Design review of the part built by this model. Coordinates are the model's own, in mm. Face numbers are marked on the shaded views. A direction names the side the tool comes from. Coordinates: 2 decimals unless noted, no trailing zeros. Order: outer loops, then holes, each group sorted by start corner. A loop starts at its lowest first (then second) coordinate and runs counter-clockwise, first axis right, second up. Notation, with made-up numbers: M -7,-19.5 L 9,-19.5 A22 ccw 9,-12.5 Z; hole C 48,-19 d7. An arc over 180 degrees is marked long. Answer as a JSON object with one key per item and string values.
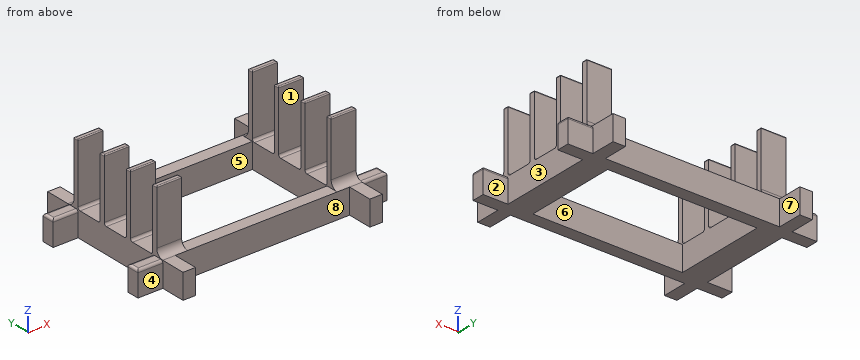
from build123d import *

# Parameters (mm, degrees)
SKETCH2_W           = 37
SKETCH2_H           = 60
BOSS_EXTRUDE1_DEPTH = 10
SKETCH3_W           = 10
SKETCH3_H           = 2
BOSS_EXTRUDE2_DEPTH = 25
FILLET1_R           = 3
FILLET2_R           = 3
FILLET3_R           = 1
FILLET6_START       = -11
FILLET6_DEPTH       = 11
FILLET6_START_2     = -43
FILLET6_2_DEPTH     = 7
FILLET6_3_DEPTH     = 11
FILLET7_START       = -11
FILLET7_DEPTH       = 11
FILLET7_START_2     = -1
FILLET7_2_DEPTH     = 7
FILLET8_R           = 1
FILLET9_R           = 1
FILLET10_R          = 0.4


with BuildPart() as part:
    # Sketch2 → Boss-Extrude1 (new body)
    with BuildSketch(Plane(origin=(0, 0, 0), x_dir=(0, 1, 0), z_dir=(0, 0, 1))):
        Polygon((-42, 10), (-42, 0), (-52, 0), (-52, -5), (-42, -5), (-42, -75), (-52, -75), (-52, -80), (-42, -80), (-42, -90), (-37, -90), (-37, -80), (0, -80), (0, -90), (5, -90), (5, -80), (15, -80), (15, -75), (5, -75), (5, -5), (15, -5), (15, 0), (5, 0), (5, 10), (0, 10), (0, 0), (-37, 0), (-37, 10), align=None)
        with Locations((-18.5, -40)):
            Rectangle(SKETCH2_W, SKETCH2_H, mode=Mode.SUBTRACT)
    extrude(amount=BOSS_EXTRUDE1_DEPTH)

    # Sketch3 → Boss-Extrude2 (add)
    with BuildSketch(Plane.XY.offset(10)):
        with Locations((5, 1)):
            Rectangle(SKETCH3_W, SKETCH3_H)
        with Locations((5, -12)):
            Rectangle(SKETCH3_W, SKETCH3_H)
        with Locations((5, -25)):
            Rectangle(SKETCH3_W, SKETCH3_H)
        with Locations((5, -38)):
            Rectangle(SKETCH3_W, SKETCH3_H)
        with Locations((75, 1)):
            Rectangle(SKETCH3_W, SKETCH3_H)
        with Locations((75, -12)):
            Rectangle(SKETCH3_W, SKETCH3_H)
        with Locations((75, -25)):
            Rectangle(SKETCH3_W, SKETCH3_H)
        with Locations((75, -38)):
            Rectangle(SKETCH3_W, SKETCH3_H)
    extrude(amount=BOSS_EXTRUDE2_DEPTH)

    # Fillet1
    fillet1_edges = [part.edges().sort_by_distance(p)[0] for p in [
        (5, -39, 10),
        (75, -39, 10),
    ]]
    fillet(fillet1_edges, radius=FILLET1_R - 0.0001)  # a hair under: the kernel refuses the full size

    # Fillet2
    fillet2_edges = [part.edges().sort_by_distance(p)[0] for p in [
        (75, 2, 10),
        (5, 2, 10),
    ]]
    fillet(fillet2_edges, radius=FILLET2_R - 0.0001)  # a hair under: the kernel refuses the full size

    # Fillet3
    # the kernel refuses this fillet: 1 mm, written as the material it adds along each edge
    with BuildSketch(Plane(origin=(80, 0, 10), x_dir=(0, -1, 0), z_dir=(-1, 0, 0)), Plane(origin=(10, -26, 10), x_dir=(0, -1, 0), z_dir=(-1, 0, 0)), Plane(origin=(10, -13, 10), x_dir=(0, -1, 0), z_dir=(-1, 0, 0)), Plane(origin=(80, -11, 10), x_dir=(0, 0, 1), z_dir=(-1, 0, 0)), Plane(origin=(80, -24, 10), x_dir=(0, 0, 1), z_dir=(-1, 0, 0)), Plane(origin=(80, -37, 10), x_dir=(0, 0, 1), z_dir=(-1, 0, 0)), Plane(origin=(10, 0, 10), x_dir=(0, -1, 0), z_dir=(-1, 0, 0))) as fillet3_piece_1:
        with BuildLine():
            CenterArc((FILLET3_R, FILLET3_R), FILLET3_R, 180, 90)
            Line((0, FILLET3_R), (0, 0))
            Line((0, 0), (FILLET3_R, 0))
        make_face()
    extrude(amount=10)
    with BuildSketch(Plane(origin=(0, -37, 10), x_dir=(0, 0, 1), z_dir=(1, 0, 0)), Plane(origin=(0, -24, 10), x_dir=(0, 0, 1), z_dir=(1, 0, 0)), Plane(origin=(0, -11, 10), x_dir=(0, 0, 1), z_dir=(1, 0, 0)), Plane(origin=(70, -13, 10), x_dir=(0, -1, 0), z_dir=(1, 0, 0)), Plane(origin=(70, -26, 10), x_dir=(0, -1, 0), z_dir=(1, 0, 0))) as fillet3_piece_2:
        with BuildLine():
            CenterArc((FILLET3_R, -FILLET3_R), FILLET3_R, 90, 90)
            Line((0, -FILLET3_R), (0, 0))
            Line((0, 0), (FILLET3_R, 0))
        make_face()
    extrude(amount=10)

    # Fillet6: read off the stored shape, not the designer's step
    # Fillet6 outline → Fillet6 (cut)
    with BuildSketch(Plane.YZ.offset(FILLET6_START)):
        with BuildLine():
            Line((-42, 10), (-42, 9))
            ThreePointArc((-42, 9), (-41.707106781, 9.707106781), (-41, 10))
            Line((-41, 10), (-42, 10))
        make_face()
    extrude(amount=FILLET6_DEPTH, mode=Mode.SUBTRACT)

    # Fillet6 2 outline → Fillet6 2 (cut)
    with BuildSketch(Plane(origin=(0, 0, 0), x_dir=(1, 0, 0), z_dir=(0, 1, 0)).offset(FILLET6_START_2)):
        with BuildLine():
            ThreePointArc((-9, -10), (-9.707106781, -9.707106781), (-10, -9))
            Line((-10, -9), (-10, -10))
            Line((-10, -10), (-9, -10))
        make_face()
    extrude(amount=FILLET6_2_DEPTH, mode=Mode.SUBTRACT)

    # Fillet6 3 outline → Fillet6 3 (cut)
    with BuildSketch(Plane.YZ.offset(FILLET6_START)):
        with BuildLine():
            ThreePointArc((-38, 10), (-37.292893219, 9.707106781), (-37, 9))
            Line((-37, 9), (-37, 10))
            Line((-37, 10), (-38, 10))
        make_face()
    extrude(amount=FILLET6_3_DEPTH, mode=Mode.SUBTRACT)

    # Fillet7: read off the stored shape, not the designer's step
    # Fillet7 outline → Fillet7 (cut)
    with BuildSketch(Plane.YZ.offset(FILLET7_START)):
        with BuildLine():
            Line((0, 10), (0, 9))
            ThreePointArc((0, 9), (0.292893219, 9.707106781), (1, 10))
            Line((1, 10), (0, 10))
        make_face()
        with BuildLine():
            Line((5, 10), (4, 10))
            ThreePointArc((4, 10), (4.707106781, 9.707106781), (5, 9))
            Line((5, 9), (5, 10))
        make_face()
    extrude(amount=FILLET7_DEPTH, mode=Mode.SUBTRACT)

    # Fillet7 2 outline → Fillet7 2 (cut)
    with BuildSketch(Plane(origin=(0, 0, 0), x_dir=(1, 0, 0), z_dir=(0, 1, 0)).offset(FILLET7_START_2)):
        with BuildLine():
            ThreePointArc((-9, -10), (-9.707106781, -9.707106781), (-10, -9))
            Line((-10, -9), (-10, -10))
            Line((-10, -10), (-9, -10))
        make_face()
    extrude(amount=FILLET7_2_DEPTH, mode=Mode.SUBTRACT)

    # Fillet8
    # the kernel refuses this fillet: 1 mm, written as the material it takes off along each edge
    with BuildSketch(Plane(origin=(80, 0, 10), x_dir=(0, 1, 0), z_dir=(1, 0, 0)), Plane(origin=(92.5, 5, 10), x_dir=(0, -1, 0), z_dir=(-1, 0, 0))) as fillet8_piece_1:
        with BuildLine():
            CenterArc((FILLET8_R, -FILLET8_R), FILLET8_R, 90, 90)
            Line((0, -FILLET8_R), (0, 0))
            Line((0, 0), (FILLET8_R, 0))
        make_face()
    extrude(amount=12.5, mode=Mode.SUBTRACT)
    with BuildSketch(Plane(origin=(90, -2.5, 10), x_dir=(-1, 0, 0), z_dir=(0, 1, 0))) as fillet8_piece_2:
        with BuildLine():
            CenterArc((FILLET8_R, -FILLET8_R), FILLET8_R, 90, 90)
            Line((0, -FILLET8_R), (0, 0))
            Line((0, 0), (FILLET8_R, 0))
        make_face()
    extrude(amount=10, mode=Mode.SUBTRACT)

    # Fillet9
    # the kernel refuses this fillet: 1 mm, written as the material it takes off along each edge
    with BuildSketch(Plane(origin=(80, -42, 10), x_dir=(0, 1, 0), z_dir=(1, 0, 0)), Plane(origin=(92.5, -37, 10), x_dir=(0, -1, 0), z_dir=(-1, 0, 0))) as fillet9_piece_1:
        with BuildLine():
            CenterArc((FILLET9_R, -FILLET9_R), FILLET9_R, 90, 90)
            Line((0, -FILLET9_R), (0, 0))
            Line((0, 0), (FILLET9_R, 0))
        make_face()
    extrude(amount=12.5, mode=Mode.SUBTRACT)
    with BuildSketch(Plane(origin=(90, -44.5, 10), x_dir=(-1, 0, 0), z_dir=(0, 1, 0))) as fillet9_piece_2:
        with BuildLine():
            CenterArc((FILLET9_R, -FILLET9_R), FILLET9_R, 90, 90)
            Line((0, -FILLET9_R), (0, 0))
            Line((0, 0), (FILLET9_R, 0))
        make_face()
    extrude(amount=10, mode=Mode.SUBTRACT)

    # Fillet10
    fillet10_edges = [part.edges().sort_by_distance(p)[0] for p in [
        (75, 0, 35),
        (80, 1, 35),
        (75, 2, 35),
        (70, 1, 35),
        (5, -37, 35),
        (0, -38, 35),
        (5, -39, 35),
        (10, -38, 35),
        (5, -24, 35),
        (0, -25, 35),
        (5, -26, 35),
        (10, -25, 35),
        (5, -11, 35),
        (0, -12, 35),
        (5, -13, 35),
        (10, -12, 35),
        (75, -11, 35),
        (70, -12, 35),
        (75, -13, 35),
        (80, -12, 35),
        (75, -24, 35),
        (70, -25, 35),
        (75, -26, 35),
        (80, -25, 35),
        (75, -37, 35),
        (70, -38, 35),
        (75, -39, 35),
        (80, -38, 35),
        (5, 0, 35),
        (10, 1, 35),
        (5, 2, 35),
        (0, 1, 35),
    ]]
    fillet(fillet10_edges, radius=FILLET10_R)


solid = part.part
1) Add section A-A (y = -30.5). State the section outline as (x, z) points, and give its area (3 significant figures).
Taken from the geometry:
{"outline": "M 0,0 L 10,0 L 10,10 L 0,10 Z; M 70,0 L 80,0 L 80,10 L 70,10 Z", "area": "200 mm2"}
2) To check wall thickness, follow L1, parallel to Y at x = 7, z = 24.5; L2, parallel to X at y = -26.5, z = 4; L3, parallel to Y at x = 25, z = 6. State the ranges of each line that lie inside material, in increasing order.
Taken from the geometry:
{"L1": "y = -39 to -37, -26 to -24, -13 to -11, 0 to 2", "L2": "x = 0 to 10, 70 to 80", "L3": "y = -42 to -37, 0 to 5"}
3) Tool access review of the marked faces 1, 2, 3, 4 and 5: name each direction out of +Z, -Z, +X, -X, +Y, -Y from which nothing blocks a thin tool from reaching the whole face with its end or side.
Taken from the geometry:
{"face 1": "+Z, +X, -X", "face 2": "+Z, -Z, +X", "face 3": "+Z, +X", "face 4": "+Z, -Z, -X, -Y", "face 5": "+Z, -Z"}
4) Add section B-B (z = 32). Count the separate pieces of the cut face and the enclosed holes in it, and give its area (3 significant figures).
Taken from the geometry:
{"separate pieces": "8", "enclosed holes": "0", "area": "160 mm2"}
5) Mouldability with a two-part tool opening along Y and no side actions: class the marked faces 6, 7 and 8 as released by +Y, released by -Y, zero draft, split by the parting line, or undercut.
Taken from the geometry:
{"face 6": "undercut", "face 7": "zero draft", "face 8": "released by -Y"}
6) Insertion check: pin 1 Ø1 at (x, y) = (64, -41) entering from +Z; pin 2 Ø1 at (x, z) = (27.5, 6.5) entering from +Y; pin 3 Ø3 at (x, z) = (23.5, 12.5) entering from -Y; pin 4 Ø5 at (x, z) = (3, 23.5) entering from +Y. Each pin has a flat end and moves straight along its axis. Give the tip position at first contact, or say it passes through.
Taken from the geometry:
{"pin 1": "stops at z = 10", "pin 2": "stops at y = 5", "pin 3": "passes through", "pin 4": "stops at y = 2"}
7) Add section C-C (x = -2.5). State the section outline as (y, z) points.
Taken from the geometry:
{"outline": "M -42,0 L -37,0 L -37,9 A1 ccw -38,10 L -41,10 A1 ccw -42,9 Z; M 0,0 L 5,0 L 5,9 A1 ccw 4,10 L 1,10 A1 ccw 0,9 Z"}
